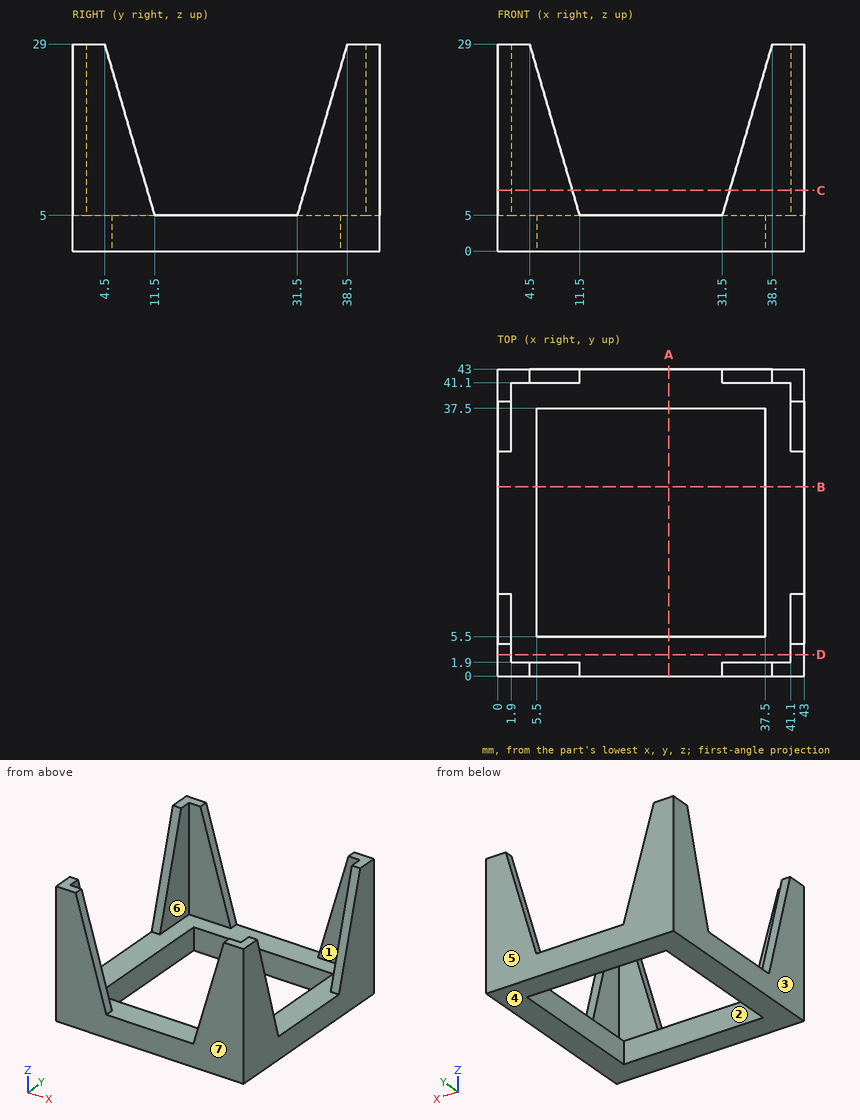
Study the drawing (mm; zero at the part's minimum x, y, z) and answer. A direction names the side the tool comes from. Give positions to 0.01 mm unless a question says otherwise; leave off trailing zeros. Loops run counter-clockwise (first coordinate to the right, second up) from the corner with the lowest first, then second, coordinate; pieces in that order, holes last. Notation, with made-up numbers: M 33.5,-24 L 54.5,-24 A7 ccw 54.5,-14 Z; hole C 75,59 d3. An arc over 180 degrees is marked long. One line per item, written item: value. Start each with the question number.
1. Find section D-D (y = 3). Give the vertices of the cut face in (x, z), and give its area (3 significant figures).
2. Determine the mould class of the marked faces 4, 5, 6 and 7 for opening direction Y: released by +Y, released by -Y, zero draft, split by the parting line, or undercut.
3. Find the intervals of material crossed by probe 1 along Y at (x, z) = (4.5, 20.5); probe 2 along Y at (x, z) = (8, 1.5), in increasing order.
4. Find section A-A (x = 24). Give the vertices of the cut face in (y, z).
5. Find section C-C (z = 8.5). Give the vertices of the cut face in (x, y), and give its area (3 significant figures).
6. Each of these flat-tipped pins is pushed along its axis until it touches: P1, Ø5, axis at x = 7, y = 5.5, coming from the -Z side; P2, Ø8, axis at x = 4.5, y = 21, coming from the +Z side. Where does it stop, or does it pass through?
7. Which of the six approach directions +Z, -Z, +X, -X, +Y, -Y give full straight-line access (tool end or side, diameter ignored) to the marked faces 1, 2 and 3?
Reported:
1. outline: M 0,0 L 43,0 L 43,29 L 41.1,29 L 41.1,5 L 1.9,5 L 1.9,29 L 0,29 Z
1. area: 306 mm²
2. face 4: zero draft
2. face 5: released by +Y
2. face 6: undercut
2. face 7: released by -Y
3. probe 1: y = 0 to 1.9, 41.1 to 43
3. probe 2: y = 0 to 5.5, 37.5 to 43
4. outline: M 0,0 L 5.5,0 L 5.5,5 L 0,5 Z; M 37.5,0 L 43,0 L 43,5 L 37.5,5 Z
5. outline: M 0,0 L 10.48,0 L 10.48,1.9 L 1.9,1.9 L 1.9,10.48 L 0,10.48 Z; M 0,32.52 L 1.9,32.52 L 1.9,41.1 L 10.48,41.1 L 10.48,43 L 0,43 Z; M 32.52,0 L 43,0 L 43,10.48 L 41.1,10.48 L 41.1,1.9 L 32.52,1.9 Z; M 32.52,41.1 L 41.1,41.1 L 41.1,32.52 L 43,32.52 L 43,43 L 32.52,43 Z
5. area: 145 mm²
6. P1: stops at z = 0
6. P2: stops at z = 5
7. face 1: +Z
7. face 2: +Z, -Z
7. face 3: +Z, -Z, -X, +Y, -Y
